Could you check a few things on this model? Use its own coordinates, in mm. A direction names the side the tool comes from. Coordinates: 2 decimals unless noted, no trailing zeros. Loops run counter-clockwise (first coordinate to the right, second up) from the corner with the lowest first, then second, coordinate; pieces in that order, holes last.
1) Imagine slicing it at D-D on z = -5. Please give me the cut outline in (x, y).
2) Imagine slicing it at A-A on y = 12. Please give me the cut outline in (x, z).
3) Thinking about a two-plate mould opening in Y: for faces 5 (the face through (9.141, -2.797, 4.447)), 6 (the face through (11, -7, 8)), 7 (the face through (4, 21, -10)), which applies, released by +Y, released by -Y, zero draft, split by the parting line, or undercut?
4) If I drill on line 1 along Y through (x, z) = (24.5, 1); line 2 along X through (y, z) = (9, -19); line 3 along X through (y, z) = (2, -25), over which ranges is the centre line in solid material (lowest first)?
5) Imagine slicing it at C-C on z = -10. Please give me the cut outline in (x, y), plus the area to 3 significant figures.
6) Will these pins go through, and if not, where does the flat tip stop? P1, Ø0.6, axis at x = 10.5, y = -14, coming from the -Z side; P2, Ø0.6, axis at x = 9.5, y = -4, coming from the -Z side; P3, Ø6.5, axis at x = 16.5, z = 6, coming from the +Y side.
7) For faces 1 (the face through (4, 6, 0)), 2 (the face through (-2.5, 3, -10)), 3 (the face through (2, 3, -8.5)), 4 (the face through (-3, 6, -10)), which set-ups out of +Z, -Z, +X, -X, +Y, -Y let a thin tool reach every point of the face, with its end or its side?
8) Imagine slicing it at B-B on z = -19. Please give me the cut outline in (x, y).
```python
from build123d import *

# Parameters (mm, degrees)
SKETCH_1_W          = 8
SKETCH_1_H          = 24
SKETCH_1_W_2        = 4
SKETCH_1_H_2        = 15
EXTRUDE_1_DEPTH     = 8
SKETCH_1_3_W        = 8
SKETCH_1_3_H        = 24
SKETCH_1_3_W_2      = 4
SKETCH_1_3_H_2      = 15
EXTRUDE_2_DEPTH     = 28
EXTRUDE_4_DEPTH     = 6
CUT_EXTRUDE_2_DEPTH = 6
SKETCH_4_W          = 8
SKETCH_4_H          = 4
EXTRUDE_5_DEPTH     = 6
FILLET_1_R          = 2
FILLET_2_R          = 3
FILLET_3_R          = 4
SKETCH_6_W          = 1.6
SKETCH_6_H          = 1.5
EXTRUDE_7_DEPTH     = 28.5
FILLET_5_R          = 0.5


with BuildPart() as part:
    # Эскиз1 → Бобышка-Вытянуть1 (new body)
    with BuildSketch(Plane.XY):
        with Locations((4, 12)):
            Rectangle(SKETCH_1_W, SKETCH_1_H)
        with Locations((4, 13.5)):
            Rectangle(SKETCH_1_W_2, SKETCH_1_H_2, mode=Mode.SUBTRACT)
    extrude(amount=EXTRUDE_1_DEPTH)

    # Эскиз1<3> → Бобышка-Вытянуть2 (add)
    with BuildSketch(Plane.XY):
        with Locations((4, 12)):
            Rectangle(SKETCH_1_3_W, SKETCH_1_3_H)
        with Locations((4, 13.5)):
            Rectangle(SKETCH_1_3_W_2, SKETCH_1_3_H_2, mode=Mode.SUBTRACT)
    extrude(amount=-EXTRUDE_2_DEPTH)

    # Эскиз3 → Бобышка-Вытянуть4 (add)
    with BuildSketch(Plane.XZ):
        with BuildLine():
            Line((0, -14), (0, -11.5))
            Line((0, -11.5), (-1, -11.5))
            ThreePointArc((-1, -11.5), (-2.5, -10), (-1, -8.5))
            Line((-1, -8.5), (0, -8.5))
            Line((0, -8.5), (0, -6))
            Line((0, -6), (-4, -6))
            Line((-4, -6), (-4, -14))
            Line((-4, -14), (0, -14))
        make_face()
    extrude(amount=-EXTRUDE_4_DEPTH)

    # Эскиз3<3> → Вырез-Вытянуть2 (cut)
    with BuildSketch(Plane.XZ):
        with BuildLine():
            Line((-1, -11.5), (0, -11.5))
            Line((0, -11.5), (0, -8.5))
            Line((0, -8.5), (-1, -8.5))
            ThreePointArc((-1, -8.5), (-2.5, -10), (-1, -11.5))
        make_face()
        with BuildLine():
            Line((0, -11.5), (5, -11.5))
            ThreePointArc((5, -11.5), (6.5, -10), (5, -8.5))
            Line((5, -8.5), (0, -8.5))
            Line((0, -8.5), (0, -11.5))
        make_face()
    extrude(amount=-CUT_EXTRUDE_2_DEPTH, mode=Mode.SUBTRACT)

    # Эскиз4 → Бобышка-Вытянуть5 (add)
    with BuildSketch(Plane.XY.offset(8)):
        Polygon((8, -4), (0, -4), (0, -19), (28.5, -19), (28.5, -4), align=None)
        with Locations((4, -2)):
            Rectangle(SKETCH_4_W, SKETCH_4_H)
    extrude(amount=-EXTRUDE_5_DEPTH)

    # Скругление1
    fillet_1_edges = [part.edges().sort_by_distance(p)[0] for p in [
        (0, 3, -14),
        (0, 3, -6),
    ]]
    fillet(fillet_1_edges, radius=FILLET_1_R)
    fillet_1_2_edges = [part.edges().sort_by_distance(p)[0] for p in [
        (-4, 3, -14),
        (-4, 3, -6),
    ]]
    fillet(fillet_1_2_edges, radius=FILLET_1_R - 0.0001)  # a hair under: the kernel refuses the full size

    # Скругление2
    fillet_2_edges = [part.edges().sort_by_distance(p)[0] for p in [
        (4, 0, 2),
    ]]
    fillet(fillet_2_edges, radius=FILLET_2_R)

    # Скругление3
    fillet_3_edges = [part.edges().sort_by_distance(p)[0] for p in [
        (8, -4, 5),
    ]]
    fillet(fillet_3_edges, radius=FILLET_3_R - 0.0001)  # a hair under: the kernel refuses the full size

    # Эскиз6 → Бобышка-Вытянуть7 (add)
    with BuildSketch(Plane(origin=(28.5, 0, 0), x_dir=(0, 0, -1), z_dir=(1, 0, 0))):
        with Locations((-1.2, -15.25)):
            Rectangle(SKETCH_6_W, SKETCH_6_H)
        with Locations((-1.2, -18.25)):
            Rectangle(SKETCH_6_W, SKETCH_6_H)
        with Locations((-1.2, -12.25)):
            Rectangle(SKETCH_6_W, SKETCH_6_H)
        with Locations((-1.2, -9.25)):
            Rectangle(SKETCH_6_W, SKETCH_6_H)
        with Locations((-1.2, -6.25)):
            Rectangle(SKETCH_6_W, SKETCH_6_H)
    extrude(amount=-EXTRUDE_7_DEPTH)

    # Скругление5
    fillet_5_edges = [part.edges().sort_by_distance(p)[0] for p in [
        (14.25, -19, 0.4),
        (14.25, -17.5, 0.4),
        (14.25, -17.5, 2),
        (14.25, -14.5, 0.4),
        (14.25, -14.5, 2),
        (14.25, -16, 2),
        (14.25, -16, 0.4),
        (14.25, -11.5, 0.4),
        (14.25, -11.5, 2),
        (14.25, -13, 2),
        (14.25, -13, 0.4),
        (14.25, -8.5, 0.4),
        (14.25, -8.5, 2),
        (14.25, -10, 2),
        (14.25, -10, 0.4),
        (14.25, -5.5, 0.4),
        (14.25, -5.5, 2),
        (14.25, -7, 2),
        (14.25, -7, 0.4),
    ]]
    fillet(fillet_5_edges, radius=FILLET_5_R)


solid = part.part
```
Filled in:
1. outline: (-0.27, 0) - (8, 0) - (8, 24) - (0, 24) - (0, 6) - (-0.27, 6) - close; hole (2, 6) - (6, 6) - (6, 21) - (2, 21) - close
2. outline: (0, -28) - (2, -28) - (2, 8) - (0, 8) - close; (6, -28) - (8, -28) - (8, 8) - (6, 8) - close
3. face 5: released by +Y
3. face 6: zero draft
3. face 7: undercut
4. line 1: y = -19 to -17.5, -16 to -14.5, -13 to -11.5, -10 to -8.5, -7 to -5.5
4. line 2: x = 0 to 2, 6 to 8
4. line 3: x = 0 to 8
5. outline: (-4, 0) - (-2.5, 0) - (-2.5, 6) - (-4, 6) - close; (0, 6) - (2, 6) - (2, 21) - (6, 21) - (6, 6) - (6.5, 6) - (6.5, 0) - (8, 0) - (8, 24) - (0, 24) - close
5. area: 102 mm2
6. P1: stops at z = 1.9
6. P2: stops at z = 2
6. P3: stops at y = -4
7. face 1: +Z, -Z
7. face 2: +Y, -Y
7. face 3: -Y
7. face 4: +Z, -Z, -X, +Y
8. outline: (0, 0) - (8, 0) - (8, 24) - (0, 24) - close; hole (2, 6) - (6, 6) - (6, 21) - (2, 21) - close
